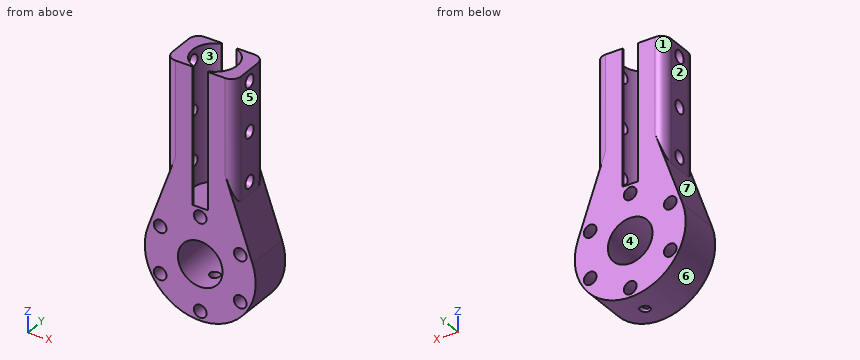
from build123d import *

# Parameters (mm, degrees)
SKETCH3_R               = 11.5
SKETCH3_R_2             = 3.2639
BOSS_EXTRUDE1_DEPTH     = 22.86
CUT_EXTRUDE1_DEPTH      = 69.85
SKETCH6_R               = 3.2639
CUT_EXTRUDE2_DEPTH      = 112.17034789
FILLET1_R               = 5
CUT_EXTRUDE4_REACH      = 97.698
CUT_EXTRUDE4_END_RADIUS = 28.575
SKETCH8_R               = 2.54


with BuildPart() as part:
    # Sketch3 → Boss-Extrude1 (new body)
    with BuildSketch(Plane(origin=(0, 0, 0), x_dir=(1, 0, 0), z_dir=(0, 1, 0))):
        with BuildLine():
            Line((-26.940768363, -9.525), (-17.78, -35.435565722))
            Line((-17.78, -35.435565722), (-17.78, -98.425))
            Line((-17.78, -98.425), (17.78, -98.425))
            Line((17.78, -98.425), (17.78, -35.435565722))
            Line((17.78, -35.435565722), (26.940768363, -9.525))
            ThreePointArc((26.940768363, -9.525), (0, 28.575), (-26.940768363, -9.525))
        make_face()
        with Locations(Location((0, 0, 0), (0, 0, 270))):
            Circle(SKETCH3_R, mode=Mode.SUBTRACT)
        with Locations(Location((0, 23.8125, 0), (0, 0, 270))):
            Circle(SKETCH3_R_2, mode=Mode.SUBTRACT)
        with Locations(Location((20.622229928, 11.90625, 0), (0, 0, 270))):
            Circle(SKETCH3_R_2, mode=Mode.SUBTRACT)
        with Locations(Location((20.622229928, -11.90625, 0), (0, 0, 270))):
            Circle(SKETCH3_R_2, mode=Mode.SUBTRACT)
        with Locations(Location((0, -23.8125, 0), (0, 0, 270))):
            Circle(SKETCH3_R_2, mode=Mode.SUBTRACT)
        with Locations(Location((-20.622229928, -11.90625, 0), (0, 0, 270))):
            Circle(SKETCH3_R_2, mode=Mode.SUBTRACT)
        with Locations(Location((-20.622229928, 11.90625, 0), (0, 0, 270))):
            Circle(SKETCH3_R_2, mode=Mode.SUBTRACT)
    extrude(amount=BOSS_EXTRUDE1_DEPTH)

    # Sketch4 → Cut-Extrude1 (cut)
    with BuildSketch(Plane.XY.offset(98.425)):
        with BuildLine():
            Line((3.96875, 0), (-3.96875, 0))
            Line((-3.96875, 0), (-3.96875, 0.583271302))
            ThreePointArc((-3.96875, 0.583271302), (-11.55, 11.43), (-3.96875, 22.276728698))
            Line((-3.96875, 22.276728698), (-3.96875, 22.86))
            Line((-3.96875, 22.86), (3.96875, 22.86))
            Line((3.96875, 22.86), (3.96875, 22.276728698))
            ThreePointArc((3.96875, 22.276728698), (11.55, 11.43), (3.96875, 0.583271302))
            Line((3.96875, 0.583271302), (3.96875, 0))
        make_face()
    extrude(amount=-CUT_EXTRUDE1_DEPTH, mode=Mode.SUBTRACT)

    # Sketch6 → Cut-Extrude2 (cut, through all)
    with BuildSketch(Plane(origin=(17.78, 0, 0), x_dir=(0, 0, -1), z_dir=(1, 0, 0))):
        with Locations((-41.785565722, 11.43)):
            Circle(SKETCH6_R)
        with Locations((-67.185565722, 11.43)):
            Circle(SKETCH6_R)
        with Locations((-92.585565722, 11.43)):
            Circle(SKETCH6_R)
    extrude(amount=-CUT_EXTRUDE2_DEPTH, mode=Mode.SUBTRACT)

    # Fillet1
    fillet1_edges = [part.edges().sort_by_distance(p)[0] for p in [
        (-17.78, 22.86, 66.930282861),
        (17.78, 22.86, 66.930282861),
        (-17.78, 0, 66.930282861),
        (17.78, 0, 66.930282861),
    ]]
    fillet(fillet1_edges, radius=FILLET1_R)

    # Cut-Extrude4: up to this cylinder (the profile starts inside it)
    cut_extrude4_end = Plane(origin=(0, 11.43, 0), z_dir=(0, -1, 0)) * Cylinder(CUT_EXTRUDE4_END_RADIUS, 253.546, mode=Mode.PRIVATE)
    # Sketch8 → Cut-Extrude4 (cut, up to the surface)
    with BuildSketch(Plane.XY.offset(10), mode=Mode.PRIVATE) as cut_extrude4_sk1:
        with Locations(Location((0, 11.43, 0), (0, 0, 90))):
            Circle(SKETCH8_R)
    cut_extrude4_tool1 = extrude(cut_extrude4_sk1.sketch, amount=-CUT_EXTRUDE4_REACH, mode=Mode.PRIVATE) & cut_extrude4_end
    add(cut_extrude4_tool1.solids().sort_by_distance((0, 11.43, 10))[0], mode=Mode.SUBTRACT)


solid = part.part
For this review, take the finished solid that the model builds, in its own axes (mm). Face numbers are marked on the shaded views. A direction names the side the tool comes from. Coordinates: 2 decimals unless noted, no trailing zeros. Loops run counter-clockwise (first coordinate to the right, second up) from the corner with the lowest first, then second, coordinate; pieces in that order, holes last. Notation, with made-up numbers: (58, -4) - (69, -4) arc R26 ccw to (69, 16) - close; hole circle Ø5 at (-10.75, 50). An arc over 180 degrees is marked (long way). Use a Markdown table: item, result. Add a question column.
Item 1: Mouldability with a two-part tool opening along Z and no side actions: class the marked faces 4, 5, 6 and 7 as pulls with the +Z half, pulls with the -Z half, needs draft (parallel to the pull), parting line crosses it, or undercut.
Item 2: Tool access review of the marked faces 1, 2 and 3: name each direction out of +Z, -Z, +X, -X, +Y, -Y from which nothing blocks a thin tool from reaching the whole face with its end or side.
Item 3: For line 1 (Y direction, x = 0, z = -14.25); line 2 (Z direction, x = -15.75, y = 11.43) (3 decimals); line 3 (Z direction, x = 13, y = 10) (3 decimals), list the stretches that pass through material, from the lowest coordinate up.
Item 4: We need section C-C (z = 56.5). Give the boundary of the cut face in (x, y).
Item 5: We need section B-B (x = 0). Give the boundary of the cut face in (y, z) (3 decimals).
Item 6: We need section D-D (y = 2.75). Give the number of separate pieces and of enclosed holes in the cut face, and give its area (3 significant figures).
Item 7: Insertion check: pin 1 Ø7 at (x, y) = (-4, 11.5) entering from +Z (3 decimals); pin 2 Ø10.5 at (y, z) = (11.43, 92.59) entering from +X; pin 3 Ø10.5 at (y, z) = (11.43, 41.79) entering from -X; pin 4 Ø6 at (y, z) = (11.43, 67.19) entering from +X. Each pin has a flat end and moves straight along its axis. Give the tip position at first contact, or say it passes through.
Item 8: We need section A-A (z = 0). Give the boundary of the cut face in (x, y) (3 decimals).
Results list:
| question | item | result |
|---|---|---|
| 1 | face 4 | undercut |
| 1 | face 5 | needs draft |
| 1 | face 6 | parting line crosses it |
| 1 | face 7 | pulls with the +Z half |
| 2 | face 1 | +Z, -X, +Y |
| 2 | face 2 | +Z, -X, +Y, -Y |
| 2 | face 3 | +Z |
| 3 | line 1 | y = 0 to 8.89, 13.97 to 22.86 |
| 3 | line 2 | z = -23.843 to 38.522, 45.049 to 63.922, 70.449 to 89.322, 95.849 to 98.425 |
| 3 | line 3 | z = -25.447 to 38.852, 44.72 to 64.252, 70.12 to 89.652, 95.52 to 98.425 |
| 4 | outline | (-17.78, 5) arc R5 ccw to (-12.78, 0) - (-3.97, 0) - (-3.97, 0.58) arc R11.55 cw to (-3.97, 22.28) - (-3.97, 22.86) - (-12.78, 22.86) arc R5 ccw to (-17.78, 17.86) - close; (3.97, 0) - (12.78, 0) arc R5 ccw to (17.78, 5) - (17.78, 17.86) arc R5 ccw to (12.78, 22.86) - (3.97, 22.86) - (3.97, 22.28) arc R11.55 cw to (3.97, 0.58) - close |
| 5 | outline | (0, -28.575) - (8.89, -28.575) - (8.89, -27.076) - (0, -27.076) - close; (0, -20.549) - (8.89, -20.549) - (8.89, -11.5) - (0, -11.5) - close; (0, 11.5) - (22.86, 11.5) - (22.86, 20.549) - (0, 20.549) - close; (0, 27.076) - (22.86, 27.076) - (22.86, 28.575) - (0, 28.575) - close; (13.97, -28.575) - (22.86, -28.575) - (22.86, -27.076) - (13.97, -27.076) - close; (13.97, -20.549) - (22.86, -20.549) - (22.86, -11.5) - (13.97, -11.5) - close |
| 6 | separate pieces | 1 |
| 6 | enclosed holes | 7 |
| 6 | area | 3,470 mm^2 |
| 7 | pin 1 | stops at z = 28.575 |
| 7 | pin 2 | stops at x = 17.78 |
| 7 | pin 3 | stops at x = -17.78 |
| 7 | pin 4 | passes through |
| 8 | outline | (-28.575, 0) - (-11.5, 0) - (-11.5, 22.86) - (-28.575, 22.86) - close; (11.5, 0) - (28.575, 0) - (28.575, 22.86) - (11.5, 22.86) - close |
